from build123d import *

# Parameters (mm, degrees)
F0_R     = 2.45
F1_DEPTH = 460
F2_DEPTH = 340


# Not quite as in the source:
# - ends of sketch curves that miss each other by under 0.0002 mm in the source are joined


with BuildPart() as f1:
    # F0 (on Front) → F1 (new body)
    with BuildSketch(Plane.XZ):
        with BuildLine():
            Line((-3.1749674082, 15), (-12, 15))
            ThreePointArc((-12, 15), (-14.1213203436, 14.1213203436), (-15, 12))
            Line((-15, 12), (-15, 3.175))
            Line((-15, 3.175), (-13.0855346263, 3.175))
            ThreePointArc((-13.0855346263, 3.175), (-12.3835980145, 3.4627605788), (-12.0856407741, 4.1604300138))
            Line((-12.0856407741, 4.1604300138), (-12.0761692778, 4.8104300138))
            ThreePointArc((-12.0761692778, 4.8104300138), (-12.3638237087, 5.5269366118), (-13.0760631299, 5.825))
            Line((-13.0760631299, 5.825), (-13.5, 5.825))
            Line((-13.5, 5.825), (-13.5, 8.225))
            Line((-13.5, 8.225), (-9.8968845016, 8.225))
            ThreePointArc((-9.8968845016, 8.225), (-9.5279915195, 8.1544718757), (-9.2111331975, 7.9528359354))
            Line((-9.2111331975, 7.9528359354), (-5.4142486959, 4.3754933338))
            ThreePointArc((-5.4142486959, 4.3754933338), (-5.1819174045, 4.0440465354), (-5.1, 3.6476573984))
            Line((-5.1, 3.6476573984), (-5.1, -3.4999243287))
            ThreePointArc((-5.1, -3.4999243287), (-5.1782354607, -3.8876744211), (-5.4007002683, -4.2147528992))
            Line((-5.4007002683, -4.2147528992), (-9.2084959767, -7.9398285705))
            ThreePointArc((-9.2084959767, -7.9398285705), (-9.5301904718, -8.1509666761), (-9.9077957084, -8.225))
            Line((-9.9077957084, -8.225), (-13.5, -8.225))
            Line((-13.5, -8.225), (-13.5, -5.825))
            Line((-13.5, -5.825), (-13.0760631299, -5.825))
            ThreePointArc((-13.0760631299, -5.825), (-12.3638237087, -5.5269366118), (-12.0761692778, -4.8104300138))
            Line((-12.0761692778, -4.8104300138), (-12.0856407741, -4.1604300138))
            ThreePointArc((-12.0856407741, -4.1604300138), (-12.3835980145, -3.4627605788), (-13.0855346263, -3.175))
            Line((-13.0855346263, -3.175), (-15, -3.175))
            Line((-15, -3.175), (-15, -12))
            ThreePointArc((-15, -12), (-14.1213203436, -14.1213203436), (-12, -15))
            Line((-12, -15), (-3.175, -15))
            Line((-3.175, -15), (-3.175, -13.0855346263))
            ThreePointArc((-3.175, -13.0855346263), (-3.4627605788, -12.3835980145), (-4.1604300138, -12.0856407741))
            Line((-4.1604300138, -12.0856407741), (-4.8104300138, -12.0761692778))
            ThreePointArc((-4.8104300138, -12.0761692778), (-5.5269366118, -12.3638237087), (-5.825, -13.0760631299))
            Line((-5.825, -13.0760631299), (-5.825, -13.5))
            Line((-5.825, -13.5), (-8.225, -13.5))
            Line((-8.225, -13.5), (-8.225, -9.8968845016))
            ThreePointArc((-8.225, -9.8968845016), (-8.1544718757, -9.5279915195), (-7.9528359354, -9.2111331975))
            Line((-7.9528359354, -9.2111331975), (-4.3754933338, -5.4142486959))
            ThreePointArc((-4.3754933338, -5.4142486959), (-4.0440465354, -5.1819174045), (-3.6476573984, -5.1))
            Line((-3.6476573984, -5.1), (3.4999243287, -5.1))
            ThreePointArc((3.4999243287, -5.1), (3.8876744211, -5.1782354607), (4.2147528992, -5.4007002683))
            Line((4.2147528992, -5.4007002683), (7.9398285705, -9.2084959767))
            ThreePointArc((7.9398285705, -9.2084959767), (8.1509666761, -9.5301904718), (8.225, -9.9077957084))
            Line((8.225, -9.9077957084), (8.225, -13.5))
            Line((8.225, -13.5), (5.825, -13.5))
            Line((5.825, -13.5), (5.825, -13.0760631299))
            ThreePointArc((5.825, -13.0760631299), (5.5269366118, -12.3638237087), (4.8104300138, -12.0761692778))
            Line((4.8104300138, -12.0761692778), (4.1604300138, -12.0856407741))
            ThreePointArc((4.1604300138, -12.0856407741), (3.4627605788, -12.3835980145), (3.175, -13.0855346263))
            Line((3.175, -13.0855346263), (3.175, -15))
            Line((3.175, -15), (12, -15))
            ThreePointArc((12, -15), (14.1213203436, -14.1213203436), (15, -12))
            Line((15, -12), (15, -3.175))
            Line((15, -3.175), (13.0855346263, -3.175))
            ThreePointArc((13.0855346263, -3.175), (12.3835980145, -3.4627605788), (12.0856407741, -4.1604300138))
            Line((12.0856407741, -4.1604300138), (12.0761692778, -4.8104300138))
            ThreePointArc((12.0761692778, -4.8104300138), (12.3638237087, -5.5269366118), (13.0760631299, -5.825))
            Line((13.0760631299, -5.825), (13.5, -5.825))
            Line((13.5, -5.825), (13.5, -8.225))
            Line((13.5, -8.225), (9.9077957084, -8.225))
            ThreePointArc((9.9077957084, -8.225), (9.5301904718, -8.1509666761), (9.2084959767, -7.9398285705))
            Line((9.2084959767, -7.9398285705), (5.4007002683, -4.2147528992))
            ThreePointArc((5.4007002683, -4.2147528992), (5.1782354607, -3.8876744211), (5.1, -3.4999243287))
            Line((5.1, -3.4999243287), (5.1, 3.6476573984))
            ThreePointArc((5.1, 3.6476573984), (5.1819174045, 4.0440465354), (5.4142486959, 4.3754933338))
            Line((5.4142486959, 4.3754933338), (9.2111331975, 7.9528359354))
            ThreePointArc((9.2111331975, 7.9528359354), (9.5279915195, 8.1544718757), (9.8968845016, 8.225))
            Line((9.8968845016, 8.225), (13.5, 8.225))
            Line((13.5, 8.225), (13.5, 5.825))
            Line((13.5, 5.825), (13.0760631299, 5.825))
            ThreePointArc((13.0760631299, 5.825), (12.3638237087, 5.5269366118), (12.0761692778, 4.8104300138))
            Line((12.0761692778, 4.8104300138), (12.0856407741, 4.1604300138))
            ThreePointArc((12.0856407741, 4.1604300138), (12.3835980145, 3.4627605788), (13.0855346263, 3.175))
            Line((13.0855346263, 3.175), (15, 3.175))
            Line((15, 3.175), (15, 12))
            ThreePointArc((15, 12), (14.1213203436, 14.1213203436), (12, 15))
            Line((12, 15), (3.1750325918, 15))
            Line((3.1750325918, 15), (3.1750325918, 13.0854824722))
            ThreePointArc((3.1750325918, 13.0854824722), (3.4627931706, 12.3835458604), (4.1604626057, 12.0855886201))
            Line((4.1604626057, 12.0855886201), (4.8104626057, 12.0761171237))
            ThreePointArc((4.8104626057, 12.0761171237), (5.5269692036, 12.3637715546), (5.8250325918, 13.0760109758))
            Line((5.8250325918, 13.0760109758), (5.8250325918, 13.4999478459))
            Line((5.8250325918, 13.4999478459), (8.2250325918, 13.4999478459))
            Line((8.2250325918, 13.4999478459), (8.2250325918, 9.8968323476))
            ThreePointArc((8.2250325918, 9.8968323476), (8.1545044675, 9.5279393654), (7.9528685272, 9.2110810434))
            Line((7.9528685272, 9.2110810434), (4.3755259256, 5.4141965418))
            ThreePointArc((4.3755259256, 5.4141965418), (4.0440791272, 5.1818652505), (3.6476899902, 5.0999478459))
            Line((3.6476899902, 5.0999478459), (-3.4998917369, 5.0999478459))
            ThreePointArc((-3.4998917369, 5.0999478459), (-3.8876418293, 5.1781833067), (-4.2147203074, 5.4006481142))
            Line((-4.2147203074, 5.4006481142), (-7.9397959787, 9.2084438226))
            ThreePointArc((-7.9397959787, 9.2084438226), (-8.1509340843, 9.5301383177), (-8.2249674082, 9.9077435543))
            Line((-8.2249674082, 9.9077435543), (-8.2249674082, 13.4999478459))
            Line((-8.2249674082, 13.4999478459), (-5.8249674082, 13.4999478459))
            Line((-5.8249674082, 13.4999478459), (-5.8249674082, 13.0760109758))
            ThreePointArc((-5.8249674082, 13.0760109758), (-5.5269040199, 12.3637715546), (-4.810397422, 12.0761171237))
            Line((-4.810397422, 12.0761171237), (-4.160397422, 12.0855886201))
            ThreePointArc((-4.160397422, 12.0855886201), (-3.462727987, 12.3835458604), (-3.1749674082, 13.0854824722))
            Line((-3.1749674082, 13.0854824722), (-3.1749674082, 15))
        make_face()
        with BuildLine():
            Line((-13.5, -11.5), (-13.5, -9.7))
            Line((-13.5, -9.7), (-9.7, -9.7))
            Line((-9.7, -9.7), (-9.7, -13.5))
            Line((-9.7, -13.5), (-11.5, -13.5))
            ThreePointArc((-11.5, -13.5), (-12.9142135624, -12.9142135624), (-13.5, -11.5))
        make_face(mode=Mode.SUBTRACT)
        with BuildLine():
            Line((9.7, -9.7), (13.5, -9.7))
            Line((13.5, -9.7), (13.5, -11.5))
            ThreePointArc((13.5, -11.5), (12.9142135624, -12.9142135624), (11.5, -13.5))
            Line((11.5, -13.5), (9.7, -13.5))
            Line((9.7, -13.5), (9.7, -9.7))
        make_face(mode=Mode.SUBTRACT)
        with BuildLine():
            ThreePointArc((-13.5, 11.5), (-12.9142135624, 12.9142135624), (-11.5, 13.5))
            Line((-11.5, 13.5), (-9.7, 13.5))
            Line((-9.7, 13.5), (-9.7, 9.7))
            Line((-9.7, 9.7), (-13.5, 9.7))
            Line((-13.5, 9.7), (-13.5, 11.5))
        make_face(mode=Mode.SUBTRACT)
        Circle(F0_R, mode=Mode.SUBTRACT)
        with BuildLine():
            Line((9.7, 13.5), (11.5, 13.5))
            ThreePointArc((11.5, 13.5), (12.9142135624, 12.9142135624), (13.5, 11.5))
            Line((13.5, 11.5), (13.5, 9.7))
            Line((13.5, 9.7), (9.7, 9.7))
            Line((9.7, 9.7), (9.7, 13.5))
        make_face(mode=Mode.SUBTRACT)
    extrude(amount=F1_DEPTH)

    # F2 (cut): a face of the model
    f2_faces = [f1.faces().sort_by_distance(p)[0] for p in [
        (5.2291627207, -460, 12.6659491494),
    ]]
    extrude(f2_faces, amount=-F2_DEPTH, mode=Mode.SUBTRACT)


solid = f1.part
Source: CAD feature listing. Evaluate the final solid. Frame: model axes, mm. A direction names the side the tool comes from. Round coordinates to 2 decimals unless told otherwise and drop trailing zeros. Order: outer loops, then holes, each group sorted by start corner. A loop starts at its lowest first (then second) coordinate and runs counter-clockwise, first axis right, second up. Notation, with made-up numbers: (68.5, 66) - (123.5, 66) arc R20 ccw to (123.5, 94) - close; hole circle Ø5 at (-17.5, -9). An arc over 180 degrees is marked (long way). Use a Markdown table: item, result. Add a question column.
1. Line query: probe 1 along Z at (x, y) = (-11, -16.5) (3 decimals); probe 2 along X at (y, z) = (-102, 4.75); probe 3 along X at (y, z) = (-10.5, -6.75). Output: solid intervals per line, ascending.
2. First-contact query: pin 1 (2 mm diameter, centred on y = -53, z = -14.5, fed in from +X); pin 2 (1.5 mm diameter, centred on x = 14, y = -60, fed in from +Z); pin 3 (1.5 mm diameter, centred on y = -46, z = -14.5, fed in from -X). Flat tips, straight axial feed; report the tip coordinate or a pass-through.
3. Section query B-B (x = 0). Return the cut outline in (y, z).
4. Set-up query: faces 4 (the flat face through (3.175, -59, 14)), 5 (the flat face through (14, -59, 3.175)), 6 (the flat face through (-7, -59, 13.5)). Return all of +Z, -Z, +X, -X, +Y, -Y with unobstructed straight access to the full face (end or side cutting, diameter ignored); none if empty.
5. Section query A-A (z = 0). Return the cut outline in (x, y), then the cut area to 3 significant figures.
6. Mould query, pull axis Z, two halves, no side actions, for faces 1 (the cylindrical face through (-0.5, -59.2, -2.4)), 2 (the cylindrical face through (14.1, -59.16, -14.14)), 3 (the flat face through (8, -59, 15)). Classes: +Z half, -Z half, draft (parallel to the pull), parting line (faces both ways), or undercut.
7. Section query C-C (y = -28). Give the number of separate pieces and of enclosed holes in the cut face, then the cut area to 3 significant figures.
Derived:
| question | item | result |
|---|---|---|
| 1 | probe 1 | -15 to -13.5, -9.7 to -8.225, 8.225 to 9.7, 13.5 to 15 |
| 1 | probe 2 | -15 to -12.08, -5.81 to 5.81, 12.08 to 15 |
| 1 | probe 3 | -15 to -13.5, -7.99 to -5.63, 5.53 to 7.99, 13.5 to 15 |
| 2 | pin 1 | x = 14.6 |
| 2 | pin 2 | z = 14.73 |
| 2 | pin 3 | x = -14.44 |
| 3 | outline | (-120, -5.1) - (0, -5.1) - (0, -2.45) - (-120, -2.45) - close; (-120, 2.45) - (0, 2.45) - (0, 5.1) - (-120, 5.1) - close |
| 4 | face 4 | +Z, +Y, -Y |
| 4 | face 5 | +X, +Y, -Y |
| 4 | face 6 | +Y, -Y |
| 5 | outline | (-5.1, -120) - (-2.45, -120) - (-2.45, 0) - (-5.1, 0) - close; (2.45, -120) - (5.1, -120) - (5.1, 0) - (2.45, 0) - close |
| 5 | area | 636 mm2 |
| 6 | face 1 | undercut |
| 6 | face 2 | -Z half |
| 6 | face 3 | +Z half |
| 7 | separate pieces | 1 |
| 7 | enclosed holes | 5 |
| 7 | area | 330 mm2 |
